```python
from build123d import *

# Parameters (mm, degrees)
CROQUIS1_R              = 4
CROQUIS1_R_2            = 2
SALIENTE_EXTRUIR1_DEPTH = 6
CROQUIS2_R              = 5
CROQUIS2_R_2            = 4
SALIENTE_EXTRUIR2_DEPTH = 19
CHAFL_N1_SIZE           = 0.3


with BuildPart() as part:
    # Croquis1 → Saliente-Extruir1 (new body)
    with BuildSketch(Plane(origin=(0, 0, 0), x_dir=(1, 0, 0), z_dir=(0, 1, 0))):
        with BuildLine():
            Line((7.549834435, 8), (-7.549834435, 8))
            ThreePointArc((-7.549834435, 8), (-11, 0), (-7.549834435, -8))
            Line((-7.549834435, -8), (7.549834435, -8))
            ThreePointArc((7.549834435, -8), (11, 0), (7.549834435, 8))
        make_face()
        with Locations(Location((0, 0, 0), (0, 0, 270))):
            Circle(CROQUIS1_R, mode=Mode.SUBTRACT)
        with Locations(Location((-8, 0, 0), (0, 0, 270))):
            Circle(CROQUIS1_R_2, mode=Mode.SUBTRACT)
        with Locations(Location((8, 0, 0), (0, 0, 270))):
            Circle(CROQUIS1_R_2, mode=Mode.SUBTRACT)
    extrude(amount=SALIENTE_EXTRUIR1_DEPTH)

    # Croquis2 → Saliente-Extruir2 (add)
    with BuildSketch(Plane(origin=(0, 6, 0), x_dir=(1, 0, 0), z_dir=(0, 1, 0))):
        with Locations(Location((0, 0, 0), (0, 0, 270))):
            Circle(CROQUIS2_R)
        with Locations(Location((0, 0, 0), (0, 0, 270))):
            Circle(CROQUIS2_R_2, mode=Mode.SUBTRACT)
    extrude(amount=SALIENTE_EXTRUIR2_DEPTH)

    # Chaflán1
    chafl_n1_edges = [part.edges().sort_by_distance(p)[0] for p in [
        (-11, 6, 0),
        (0, 0, -4),
        (0, 6, 8),
        (-8, 0, -2),
        (-8, 6, -2),
        (8, 0, -2),
        (8, 6, -2),
        (0, 25, -5),
        (0, 6, -5),
        (0, 25, -4),
        (11, 6, 0),
        (0, 0, 8),
        (-11, 0, 0),
        (0, 0, -8),
        (11, 0, 0),
        (0, 6, -8),
    ]]
    chamfer(chafl_n1_edges, length=CHAFL_N1_SIZE)


solid = part.part
```
The listing builds one solid part. Answer for the finished solid, in the listing's coordinates (mm). A direction names the side the tool comes from. Coordinates: 2 decimals unless noted, no trailing zeros. Write each loop counter-clockwise with the first axis right and the second up, starting at its lowest first coordinate (ties: lowest second). Pieces come first, ordered by that corner, then holes. Notation, with made-up numbers: (26, -2) - (56, -2) arc R8 cw to (56, 3) - close; hole circle Ø9 at (27.25, 27). An arc over 180 degrees is marked (long way). Return JSON: item names as keys, results as strings. Group by question number.
Q1. Flat-ended cylindrical pins translate along their axes: pin 1 Ø4 at (x, y) = (-1, 14) entering from +Z; pin 2 Ø8 at (x, y) = (4.5, 21) entering from -Z; pin 3 Ø4 at (y, z) = (19, -1.5) entering from +X. Find the tip coordinate at first contact, or state that the pin passes through.
Q2. Find the intervals of material crossed by line 1 along X through (y, z) = (4.2, 0); line 2 along X through (y, z) = (22.25, 0); line 3 along Y through (x, z) = (-5, 2.5), in increasing order. Write a range as [from, to].
Q3. The part is cut by section A-A on y = 20.5. Write down the section's boundary in (x, z), and give its area (3 significant figures).
Q4. The part is cut by section B-B on z = 0. State how many separate pieces and enclosed holes the cut face has, and give its area (3 significant figures).
Q5. Which of the six approach directions +Z, -Z, +X, -X, +Y, -Y give full straight-line access (tool end or side, diameter ignored) to faces 5 (the flat face through (0, 3, 8)), 6 (the flat face through (-3, 6, 5))?
Q6. For a pull along X with two mould halves and no side action, classify faces 1 (the cylindrical face through (-11, 3, 0)), 2 (the flat face through (-4, 25, 2)), 3 (the cylindrical face through (11, 3, 0)), 4 (the cylindrical face through (10, 3, 0)) as +X half, -X half, draft (parallel to the pull), parting line (faces both ways), or undercut.
Evaluation:
{
 "1": {"pin 1": "stops at z = 5", "pin 2": "stops at z = -4.97", "pin 3": "stops at x = 5"},
 "2": {"line 1": "x = [-11, -10], [-6, -4], [4, 6], [10, 11]", "line 2": "x = [-5, -4], [4, 5]", "line 3": "y = [0, 6]"},
 "3": {"outline": "circle Ø10 at (0, 0); hole circle Ø8 at (0, 0)", "area": "28.3 mm2"},
 "4": {"separate pieces": "4", "enclosed holes": "0", "area": "73.3 mm2"},
 "5": {"face 5": "+Z, +X, -X, +Y, -Y", "face 6": "+Y"},
 "6": {"face 1": "-X half", "face 2": "draft", "face 3": "+X half", "face 4": "undercut"}
}
